Input: part model. Units: mm. Frame: model coordinates. Coordinates: 2 decimals unless noted, no trailing zeros. Write each loop counter-clockwise with the first axis right and the second up, starting at its lowest first coordinate (ties: lowest second). Pieces come first, ordered by that corner, then holes.
1) Line query: L1, parallel to X at y = -46.5, z = 0; L2, parallel to X at y = -42, z = 15; L3, parallel to Z at x = -16.5, y = -45. Output: solid intervals per line, ascending.
2) Pin query (flat end, axial travel): pin 1 Ø1 at (x, y) = (-22, -47.5) entering from +Z; pin 2 Ø12 at (x, z) = (-13.5, 17.5) entering from +Y; pin 3 Ø6 at (x, z) = (12.5, 4.5) entering from -Y; pin 4 Ø1.5 at (x, y) = (-23, -4.5) entering from -Z. Return the tip coordinate at first contact, or that it passes through.
3) Draft query along Z for faces 1 (the cylindrical face through (10.363, -44.415, -32.907)), 2 (the cylindrical face through (-9.76, -44.09, -31)). Return one class per face: pulls with the +Z half, pulls with the -Z half, needs draft (parallel to the pull), parting line crosses it, or undercut.
4) Section query C-C (y = -25.5). Output: boundary loops of the cut face in (x, z), then the cut area to 3 significant figures.
Autodesk Inventor part; units mm, degrees
ref_plane "YZ Plane" through (0, 0, 0) normal (1, 0, 0) x (0, 1, 0)
ref_plane "XZ Plane" through (0, 0, 0) normal (0, 1, 0) x (-1, 0, 0)
ref_plane "XY Plane" through (0, 0, 0) normal (0, 0, 1) x (1, 0, 0)
sketch "Sketch1" plane through (0, 0, 0) normal (1, 0, 0) x (0, 1, 0)
  line L0 (0, 0) -> (-57, 0)
  line L1 (0, 0) -> (2, 0)
  line L2 (-57, 0) -> (-57, -32.5)
  line L3 (-57, -32.5) -> (-57, -34.5)
  line L4 (0, 0) -> (-32.5, 0)
  circle A0 centre (-32.5, 0) radius 32.5
  circle A1 centre (-32.5, 0) radius 34.5
  line L5 (-57, -32.5) -> (-32.5, -32.5)
  line L6 (-32.5, -34.5) -> (-57, -34.5)
  line L7 (0, 0) -> (2, 0)
  dimension "d0" = 57
  dimension "d1" = 2
  dimension "d2" = 32.5
  dimension "d3" = 2
  dimension "d4" = 32.5
revolve "Revolution1" add sketch "Sketch1" angle 360 about axis through (0, 0, 0) along (0, -1, 0) contours L1 A1 L5 A0 | L6 L3 L5 A1
fillet "Fillet1" radius 1 1 edges at (0, -57, 34.5)
fillet "Fillet2" radius 1 1 edges at (0, -57, 32.5)
properties part number "BlueYetiCap"
Answer:
1. L1: x = -34.5 to -32.5, 32.5 to 34.5
1. L2: x = -31.07 to -28.83, 28.83 to 31.07
1. L3: z = -30.3 to -28, 28 to 30.3
2. pin 1: stops at z = 26.98
2. pin 2: stops at y = -1.99
2. pin 3: stops at y = -4.37
2. pin 4: passes through
3. face 1: parting line crosses it
3. face 2: undercut
4. outline: circle Ø67.56 at (0, 0); hole circle Ø63.47 at (0, 0)
4. area: 421 mm2
